from build123d import *

# Parameters (mm, degrees)
SKETCH1_W           = 57.4
SKETCH1_H           = 33
SKETCH1_R           = 1.65
BOSS_EXTRUDE1_DEPTH = 1
CUT_EXTRUDE1_REACH  = 68.218
SKETCH2_W           = 57.4
SKETCH2_H           = 2.3
BOSS_EXTRUDE2_DEPTH = 57.4
FILLET1_R           = 2
BOSS_EXTRUDE3_DEPTH = 57.4
SKETCH4_R           = 1.65
CUT_EXTRUDE2_DEPTH  = 2
CUT_EXTRUDE3_REACH  = 67.163
SKETCH5_R           = 2.75
SKETCH6_R           = 1.15
CUT_EXTRUDE4_DEPTH  = 3
SKETCH9_R           = 2.5
CUT_EXTRUDE5_DEPTH  = 64.930040028
FILLET2_R           = 2


with BuildPart() as part:
    # Sketch1 → Boss-Extrude1 (new body)
    with BuildSketch(Plane(origin=(0, 0, 0), x_dir=(1, 0, 0), z_dir=(0, 1, 0))):
        with Locations((28.7, 16.5)):
            Rectangle(SKETCH1_W, SKETCH1_H)
        with Locations(Location((4.5, 28.3, 0), (0, 0, 270))):
            Circle(SKETCH1_R, mode=Mode.SUBTRACT)
        with Locations(Location((51.5, 28.3, 0), (0, 0, 270))):
            Circle(SKETCH1_R, mode=Mode.SUBTRACT)
        with Locations(Location((4.5, 4.7, 0), (0, 0, 270))):
            Circle(SKETCH1_R, mode=Mode.SUBTRACT)
        with Locations(Location((51.5, 4.7, 0), (0, 0, 270))):
            Circle(SKETCH1_R, mode=Mode.SUBTRACT)
    extrude(amount=BOSS_EXTRUDE1_DEPTH)

    # Sketch2 → Cut-Extrude1 (cut, up to next)
    with BuildSketch(Plane(origin=(0, 1, 0), x_dir=(1, 0, 0), z_dir=(0, 1, 0)), mode=Mode.PRIVATE) as cut_extrude1_sk1:
        with Locations((28.7, 31.85)):
            Rectangle(SKETCH2_W, SKETCH2_H)
    cut_extrude1_tool1 = extrude(cut_extrude1_sk1.sketch, amount=-CUT_EXTRUDE1_REACH, mode=Mode.PRIVATE) & part.part
    add(cut_extrude1_tool1.solids().sort_by_distance((28.7, 1, -31.85))[0], mode=Mode.SUBTRACT)

    # Sketch3 → Boss-Extrude2 (add)
    with BuildSketch(Plane(origin=(57.4, 0, 0), x_dir=(0, 0, -1), z_dir=(1, 0, 0))):
        Polygon((30.7, 1), (30.7, 5), (28.7, 5), (20.7, 1), align=None)
    extrude(amount=-BOSS_EXTRUDE2_DEPTH)

    # Fillet1
    fillet1_edges = [part.edges().sort_by_distance(p)[0] for p in [
        (57.4, 0.5, 0),
        (0, 0.5, 0),
    ]]
    fillet(fillet1_edges, radius=FILLET1_R)

    # Sketch10 → Boss-Extrude3 (add)
    with BuildSketch(Plane(origin=(0, 0, 0), x_dir=(0, 0, -1), z_dir=(1, 0, 0))):
        with BuildLine():
            Line((0, 1), (2, 1))
            Line((2, 1), (20.7, 1))
            Line((20.7, 1), (28.7, 5))
            Line((28.7, 5), (28.668697288, 5))
            ThreePointArc((28.668697288, 5), (14.522580868, 1.323329002), (0, 2.974136187))
            Line((0, 2.974136187), (0, 1))
        make_face()
    extrude(amount=BOSS_EXTRUDE3_DEPTH)

    # Sketch4 → Cut-Extrude2 (cut)
    with BuildSketch(Plane(origin=(0, 0, 0), x_dir=(-1, 0, 0), z_dir=(0, -1, 0))):
        with Locations(Location((-4.5, 28.3, 0), (0, 0, 90))):
            Circle(SKETCH4_R)
        with Locations(Location((-51.5, 28.3, 0), (0, 0, 90))):
            Circle(SKETCH4_R)
    extrude(amount=-CUT_EXTRUDE2_DEPTH, mode=Mode.SUBTRACT)

    # Sketch5 → Cut-Extrude3 (cut, up to next)
    with BuildSketch(Plane(origin=(0, 2, 0), x_dir=(-1, 0, 0), z_dir=(0, -1, 0)), mode=Mode.PRIVATE) as cut_extrude3_sk1:
        with Locations((-4.5, 28.3)):
            Circle(SKETCH5_R)
    cut_extrude3_tool1 = extrude(cut_extrude3_sk1.sketch, amount=-CUT_EXTRUDE3_REACH, mode=Mode.PRIVATE) & part.part
    # Sketch5 → Cut-Extrude3 (cut, up to next)
    with BuildSketch(Plane(origin=(0, 2, 0), x_dir=(-1, 0, 0), z_dir=(0, -1, 0)), mode=Mode.PRIVATE) as cut_extrude3_sk2:
        with Locations((-51.5, 28.3)):
            Circle(SKETCH5_R)
    cut_extrude3_tool2 = extrude(cut_extrude3_sk2.sketch, amount=-CUT_EXTRUDE3_REACH, mode=Mode.PRIVATE) & part.part
    add(cut_extrude3_tool1.solids().sort_by_distance((4.5, 2, -28.3))[0], mode=Mode.SUBTRACT)
    add(cut_extrude3_tool2.solids().sort_by_distance((51.5, 2, -28.3))[0], mode=Mode.SUBTRACT)

    # Sketch6 → Cut-Extrude4 (cut)
    with BuildSketch(Plane(origin=(0, 0, -30.7), x_dir=(-1, 0, 0), z_dir=(0, 0, -1))):
        with Locations((-38.7, 3)):
            Circle(SKETCH6_R)
        with Locations((-18.7, 3)):
            Circle(SKETCH6_R)
    extrude(amount=-CUT_EXTRUDE4_DEPTH, mode=Mode.SUBTRACT)

    # Sketch9 → Cut-Extrude5 (cut, through all)
    with BuildSketch(Plane(origin=(0, 0, -27.7), x_dir=(-1, 0, 0), z_dir=(0, 0, -1))):
        with Locations((-38.7, 3)):
            Circle(SKETCH9_R)
        with Locations((-18.7, 3)):
            Circle(SKETCH9_R)
    extrude(amount=-CUT_EXTRUDE5_DEPTH, mode=Mode.SUBTRACT)

    # Fillet2
    fillet2_edges = [part.edges().sort_by_distance(p)[0] for p in [
        (0, 1.987068094, 0),
        (57.4, 1.987068094, 0),
    ]]
    fillet(fillet2_edges, radius=FILLET2_R)


solid = part.part
For this review, take the finished solid that the model builds, in its own axes (mm). A direction names the side the tool comes from. Round coordinates to 2 decimals unless told otherwise and drop trailing zeros. Write each loop counter-clockwise with the first axis right and the second up, starting at its lowest first coordinate (ties: lowest second). Pieces come first, ordered by that corner, then holes. Notation, with made-up numbers: M 34,66.5 L 45,66.5 A26 cw 45,80.5 Z; hole C 26,71.25 d5. An arc over 180 degrees is marked long. Write item = value, one per line. Start each with the question number.
(1) For faces 4 (the face through (3.868, 0.493, -3.176)), 5 (the face through (38.7, 1.7, -27.7)), 6 (the face through (51.6, 3.15, -25.55)), 7 (the face through (56.8, 0.51, -0.57)), list the 3-axis set-ups (+Z, -Z, +X, -X, +Y, -Y) from which the entire face can be reached by the end or side of a thin tool; tool diameter is ignored.
(2) We need section A-A (x = 38.7). Give the boundary of the cut face in (y, z), then the cut area to 3 significant figures.
(3) We need section B-B (z = -21). Give the boundary of the cut face in (x, y), then the cut area to 3 significant figures.
(4) We need section D-D (z = -4). Give the boundary of the cut face in (x, y).
(5) The part is to be moulded in two halves that separate along Y. For faces 1 (the face through (28, 5, -30)), 2 (the face through (18.7, 1.7, -27.7)), 3 (the face through (28, 0, -16)), say which applies: +Y half, -Y half, draft (parallel to the pull), parting line (faces both ways), or undercut.
(6) Clearance check with flat-ended pins moving along their axes: pin 1 Ø3 at (x, y) = (18, 2.5) entering from +Z; pin 2 Ø1 at (x, z) = (4, -4) entering from -Y; pin 3 Ø4.5 at (x, z) = (4.5, -28.3) entering from +Y. State where each tip first meets the part, or that it passes through.
(7) We need section C-C (z = -13). Give the boundary of the cut face in (x, y), then the cut area to 3 significant figures.
(8) For line 1 along X through (y, z) = (4.4, -28.5); line 2 along X through (y, z) = (0.45, -4.7); line 3 along Y through (x, z) = (38.7, -29.75), list the stretches that pass through material, from the lowest coordinate up.
Results found:
q1.face_4 = -Y
q1.face_5 = +Z
q1.face_6 = +Y
q1.face_7 = +Z, +X, +Y, -Y
q2.outline = M 0,-30.7 L 1.85,-30.7 L 1.85,-27.7 L 0.5,-27.7 L 0.5,0 L 0,0 Z; M 4.15,-30.7 L 5,-30.7 L 5,-28.67 A40 cw 4.56,-27.7 L 4.15,-27.7 Z
q2.area = 21.7 mm²
q3.outline = M 0,0 L 57.4,0 L 57.4,2.32 L 41.11,2.32 A2.5 cw 36.29,2.32 L 21.11,2.32 A2.5 cw 16.29,2.32 L 0,2.32 Z
q3.area = 120 mm²
q4.outline = M 0,0 L 3.01,0 L 3.01,1 L 5.99,1 L 5.99,0 L 50.01,0 L 50.01,1 L 52.99,1 L 52.99,0 L 57.4,0 L 57.4,1.97 L 40.98,1.97 A2.5 cw 36.42,1.97 L 20.98,1.97 A2.5 cw 16.42,1.97 L 0,1.97 Z
q5.face_1 = +Y half
q5.face_2 = undercut
q5.face_3 = -Y half
q6.pin_1 = -27.7
q6.pin_2 = 1
q6.pin_3 = 2
q7.outline = M 0,0 L 57.4,0 L 57.4,1.24 L 40.48,1.24 A2.5 cw 36.92,1.24 L 20.48,1.24 A2.5 cw 16.92,1.24 L 0,1.24 Z
q7.area = 67.8 mm²
q8.line_1 = 0 to 1.76, 7.24 to 48.76, 54.24 to 57.4
q8.line_2 = 0 to 2.85, 6.15 to 49.85, 53.15 to 57.4
q8.line_3 = 0 to 1.85, 4.15 to 5
